Design review of the part built by this model. Coordinates are the model's own, in mm. Face numbers are marked on the shaded views. A direction names the side the tool comes from. Round coordinates to 2 decimals unless told otherwise and drop trailing zeros. Loops run counter-clockwise (first coordinate to the right, second up) from the corner with the lowest first, then second, coordinate; pieces in that order, holes last. Notation, with made-up numbers: M -15.5,71 L 34.5,71 A26 ccw 34.5,108 Z; hole C 10.25,0.5 d7. An arc over 180 degrees is marked long. One line per item, written item: value. Start each with the question number.
Item 1: We need section B-B (z = 3.25). Write out the cut boundary in (x, y).
Item 2: For line 1 along Z through (x, y) = (-1, 0.5); line 2 along X through (y, z) = (15, 9.5); line 3 along Y through (x, z) = (-49, 12.75), list the stretches that pass through material, from the lowest coordinate up.
Item 3: We need section C-C (y = 8). Write out the cut boundary in (x, z).
Item 4: We need section A-A (x = -5.5). Write out the cut boundary in (y, z).
Item 5: Clearance check with flat-ended pins moving along their axes: pin 1 (12.5 mm diameter, centred on y = 4, z = 14.5, fed in from +X); pin 2 (7 mm diameter, centred on x = 3, y = 18.5, fed in from +Z); pin 3 (2 mm diameter, centred on y = 17.5, z = 10, fed in from -X); pin 4 (10 mm diameter, centred on y = 8, z = 22.5, fed in from +X). State where each tip first meets the part, or that it passes through.
Item 6: We need section D-D (x = -39). Write out the cut boundary in (y, z), then the cut area to 3 significant figures.
Item 7: For the marked faces 5, 6 and 7, list the 3-axis set-ups (+Z, -Z, +X, -X, +Y, -Y) from which the entire face can be reached by the end or side of a thin tool; tool diameter is ignored.
Item 8: Mouldability with a two-part tool opening along Z and no side actions: class the marked faces 1, 2, 3 and 4 as released by +Z, released by -Z, zero draft, split by the parting line, or undercut.
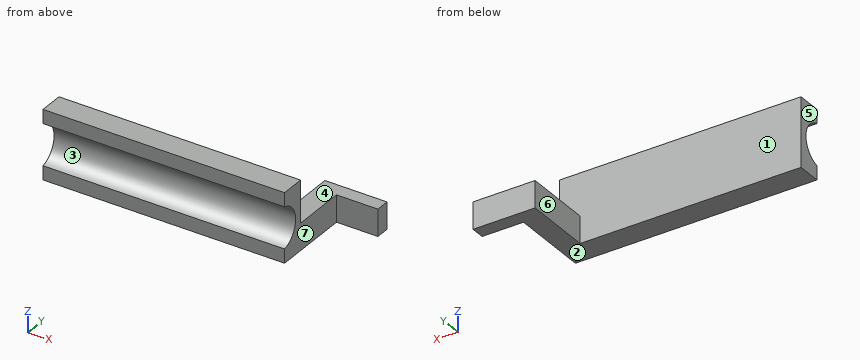
from build123d import *

# Parameters (mm, degrees)
F0_W     = 88.9
F0_H     = 25.4
F1_DEPTH = 8.89
F2_R     = 7.75
F3_DEPTH = 88.901
F4_W     = 7.62
F4_H     = 9.8552
F5_DEPTH = 25.0952
F6_W     = 5.08
F6_H     = 9.8552
F7_DEPTH = 15.24


with BuildPart() as f1:
    # F0 (on Front) → F1 (new body)
    with BuildSketch(Plane.XZ):
        with Locations((-44.45, 12.7)):
            Rectangle(F0_W, F0_H)
    extrude(amount=F1_DEPTH)

    # F2 (on face) → F3 (cut, through all)
    with BuildSketch(Plane(origin=(-88.9, 0, 0), x_dir=(0, -1, 0), z_dir=(-1, 0, 0))):
        with Locations((10.4775, 12.7)):
            Circle(F2_R)
    extrude(amount=-F3_DEPTH, mode=Mode.SUBTRACT)

    # F4 (on face) → F5 (join)
    with BuildSketch(Plane(origin=(0, 0, 0), x_dir=(-1, 0, 0), z_dir=(0, 1, 0))):
        with Locations((3.81, 4.9276)):
            Rectangle(F4_W, F4_H)
    extrude(amount=F5_DEPTH)

    # F6 (on face) → F7 (join)
    with BuildSketch(Plane.YZ):
        with Locations((22.5552, 4.9276)):
            Rectangle(F6_W, F6_H)
    extrude(amount=F7_DEPTH)


solid = f1.part
A:
1. outline: M -88.9,-8.89 L 0,-8.89 L 0,20.02 L 15.24,20.02 L 15.24,25.1 L -7.62,25.1 L -7.62,0 L -88.9,0 Z
2. line 1: 0 to 9.86
2. line 2: -7.62 to 0
2. line 3: -2.73 to 0
3. outline: M -7.62,0 L 0,0 L 0,9.86 L -7.62,9.86 Z
4. outline: M -8.89,0 L 25.1,0 L 25.1,9.86 L 0,9.86 L 0,25.4 L -8.89,25.4 L -8.89,20.29 A7.75 cw -8.89,5.11 Z
5. pin 1: x = 0
5. pin 2: z = 9.86
5. pin 3: x = -7.62
5. pin 4: through
6. outline: M -8.89,0 L 0,0 L 0,25.4 L -8.89,25.4 L -8.89,20.29 A7.75 cw -8.89,5.11 Z
6. area: 156 mm2
7. face 5: +Z, -Z, -X, +Y, -Y
7. face 6: +Z, -Z, -X, +Y
7. face 7: +Z, -Z, +X, -Y
8. face 1: zero draft
8. face 2: released by -Z
8. face 3: undercut
8. face 4: released by +Z
